Here's how the part is built. I have some questions about the finished solid (model axes, mm). Round coordinates to 2 decimals unless told otherwise and drop trailing zeros. Loops run counter-clockwise (first coordinate to the right, second up) from the corner with the lowest first, then second, coordinate; pieces in that order, holes last. Notation, with made-up numbers: M -6.5,72 L 34.5,72 A26 cw 34.5,92 Z; hole C 88,-2.75 d2. An arc over 180 degrees is marked long. Write each question's results on one line, items separated by ' | '. Start each with the question number.
```python
from build123d import *

# Parameters (mm, degrees)
CROQUIS1_W              = 140
CROQUIS1_H              = 275
SALIENTE_EXTRUIR1_DEPTH = 2.5
CROQUIS2_W              = 42
CROQUIS2_H              = 36
SALIENTE_EXTRUIR2_DEPTH = 1
CROQUIS3_W              = 140
CROQUIS3_H              = 60
CORTAR_EXTRUIR1_DEPTH   = 4.5


with BuildPart() as part:
    # Croquis1 → Saliente-Extruir1 (new body)
    with BuildSketch(Plane(origin=(0, 0, 0), x_dir=(1, 0, 0), z_dir=(0, 1, 0))):
        Rectangle(CROQUIS1_W, CROQUIS1_H)
    extrude(amount=SALIENTE_EXTRUIR1_DEPTH)

    # Croquis2 → Saliente-Extruir2 (add)
    with BuildSketch(Plane(origin=(0, 0, 0), x_dir=(-1, 0, 0), z_dir=(0, -1, 0))):
        with Locations((35, 0)):
            Rectangle(CROQUIS2_W, CROQUIS2_H)
        with Locations((-35, 0)):
            Rectangle(CROQUIS2_W, CROQUIS2_H)
    extrude(amount=SALIENTE_EXTRUIR2_DEPTH)

    # Croquis3 → Cortar-Extruir1 (cut, through all)
    with BuildSketch(Plane(origin=(0, 2.5, 0), x_dir=(1, 0, 0), z_dir=(0, 1, 0))):
        with Locations((0, 107.5)):
            Rectangle(CROQUIS3_W, CROQUIS3_H)
    extrude(amount=-CORTAR_EXTRUIR1_DEPTH, mode=Mode.SUBTRACT)


solid = part.part
```
Item 1: If we section it at B-B on z = -5.5: Please give me the cut outline in (x, y).
Item 2: If we section it at A-A on x = -45.5: Please give me the cut outline in (y, z), and give its area (4 significant figures).
Item 3: If we section it at C-C on z = 37.5: Please give me the cut outline in (x, y).
Item 4: If we section it at D-D on x = 9: Please give me the cut outline in (y, z), and give its area (4 significant figures).
Item 5: I'm going to push flat-ended pins straight in: pin 1 (1.1 mm diameter, centred on x = 39, y = -0.5, fed in from +Z); pin 2 (10 mm diameter, centred on x = -50.5, z = 47, fed in from -Y); pin 3 (0.5 mm diameter, centred on x = -33.5, y = -0.5, fed in from +Z); pin 4 (0.8 mm diameter, centred on y = -0.5, z = 4.5, fed in from +X). Where does each tip first touch, or does it pass through?
Item 6: I need wall thicknesses on L1, parallel to Z at x = 17, y = -0.4; L2, parallel to Y at x = -30, z = 102.5. Which ranges of each line are inside material? Lowest first, please.
Numbers:
1) outline: M -70,0 L -56,0 L -56,-1 L -14,-1 L -14,0 L 14,0 L 14,-1 L 56,-1 L 56,0 L 70,0 L 70,2.5 L -70,2.5 Z
2) outline: M -1,-18 L 0,-18 L 0,-77.5 L 2.5,-77.5 L 2.5,137.5 L 0,137.5 L 0,18 L -1,18 Z | area: 573.5 mm²
3) outline: M -70,0 L 70,0 L 70,2.5 L -70,2.5 Z
4) outline: M 0,-77.5 L 2.5,-77.5 L 2.5,137.5 L 0,137.5 Z | area: 537.5 mm²
5) pin 1: z = 137.5 | pin 2: y = 0 | pin 3: z = 18 | pin 4: x = 56
6) L1: -18 to 18 | L2: 0 to 2.5
